from build123d import *

# Parameters (mm, degrees)
F0_W     = 44.359287
F0_H     = 73.47857
F1_DEPTH = 12.7


with BuildPart() as f1:
    # F0 (on Top) → F1 (new body)
    with BuildSketch(Plane.XY):
        with BuildLine():
            ThreePointArc((23.268217, 27.350357), (1.088574, 49.53), (-21.09107, 27.350357))
            Line((-21.09107, 27.350357), (23.268217, 27.350357))
        make_face()
        with Locations((1.088574, -9.388928)):
            Rectangle(F0_W, F0_H)
        with BuildLine():
            Line((23.268217, -46.128213), (-21.09107, -46.128213))
            ThreePointArc((-21.09107, -46.128213), (1.088574, -68.307857), (23.268217, -46.128213))
        make_face()
    extrude(amount=F1_DEPTH)


solid = f1.part
Could you check a few things on this model? Use its own coordinates, in mm. Give positions to 0.01 mm unless a question says otherwise; leave off trailing zeros. Order: outer loops, then holes, each group sorted by start corner. A loop starts at its lowest first (then second) coordinate and runs counter-clockwise, first axis right, second up.
Item 1: If we section it at A-A, the plane z = 3.25: Write out the boundary of the cut face in (x, y).
Item 2: I need wall thicknesses on line 1 (Y direction, x = 0.5, z = 8); line 2 (Y direction, x = 14, z = 2.5); line 3 (X direction, y = 38, z = 5.25). Which ranges of each line are inside material? Lowest first, please.
Item 3: I'm going to push flat-ended pins straight in: pin 1 (1.5 mm diameter, centred on y = 36, z = 5.5, fed in from +X); pin 2 (5 mm diameter, centred on x = 8.5, z = 7.5, fed in from +Y); pin 3 (5 mm diameter, centred on x = -0.5, z = 5, fed in from -Y). Where does each tip first touch, or does it pass through?
Item 4: If we section it at B-B, the plane x = 12: Write out the boundary of the cut face in (y, z).
Values:
1. outline: (-21.09, -46.13) arc R22.18 ccw to (23.27, -46.13) - (23.27, 27.35) arc R22.18 ccw to (-21.09, 27.35) - close
2. line 1: y = -68.3 to 49.52
2. line 2: y = -64.16 to 45.38
2. line 3: x = -18.37 to 20.54
3. pin 1: stops at x = 21.81
3. pin 2: stops at y = 48.98
3. pin 3: stops at y = -68.31
4. outline: (-65.44, 0) - (46.66, 0) - (46.66, 12.7) - (-65.44, 12.7) - close
